from build123d import *

# Parameters (mm, degrees)
BOSS_EXTRUDE1_DEPTH                 = 90
CUT_EXTRUDE1_REACH                  = 116.455
CUT_EXTRUDE2_REACH                  = 116.455
CUT_EXTRUDE2_END_RADIUS             = 50
SKETCH3_W                           = 40
SKETCH3_H                           = 20
CUT_EXTRUDE2_DIRECTION_2_REACH      = 116.455
CUT_EXTRUDE2_DIRECTION_2_END_RADIUS = 50


with BuildPart() as part:
    # Sketch1 → Boss-Extrude1 (new body)
    with BuildSketch(Plane(origin=(0, 0, 0), x_dir=(0, 0, -1), z_dir=(1, 0, 0))):
        with BuildLine():
            Line((-50, 0), (50, 0))
            ThreePointArc((50, 0), (0, 50), (-50, 0))
        make_face()
    extrude(amount=BOSS_EXTRUDE1_DEPTH)

    # Sketch2 → Cut-Extrude1 (cut, up to next)
    with BuildSketch(Plane.ZY, mode=Mode.PRIVATE) as cut_extrude1_sk1:
        Polygon((0, 20.207259422), (-17.5, 10.103629711), (-17.5, -10.103629711), (0, -20.207259422), (17.5, -10.103629711), (17.5, 10.103629711), align=None)
    cut_extrude1_tool1 = extrude(cut_extrude1_sk1.sketch, amount=-CUT_EXTRUDE1_REACH, mode=Mode.PRIVATE) & part.part
    add(cut_extrude1_tool1.solids().sort_by_distance((0, 0, 0))[0], mode=Mode.SUBTRACT)

    # Cut-Extrude2: up to this cylinder (the profile starts inside it)
    cut_extrude2_end = Plane(origin=(45, 0, 0), z_dir=(-1, 0, 0)) * Cylinder(CUT_EXTRUDE2_END_RADIUS, 333.91, mode=Mode.PRIVATE)
    # Sketch3 → Cut-Extrude2 (cut, up to the surface)
    with BuildSketch(Plane.XY, mode=Mode.PRIVATE) as cut_extrude2_sk1:
        with Locations((45, 40)):
            Rectangle(SKETCH3_W, SKETCH3_H)
    cut_extrude2_tool1 = extrude(cut_extrude2_sk1.sketch, amount=-CUT_EXTRUDE2_REACH, mode=Mode.PRIVATE) & cut_extrude2_end
    add(cut_extrude2_tool1.solids().sort_by_distance((45, 40, 0))[0], mode=Mode.SUBTRACT)

    # Cut-Extrude2 direction 2: up to this cylinder (the profile starts inside it)
    cut_extrude2_direction_2_end = Plane(origin=(45, 0, 0), z_dir=(-1, 0, 0)) * Cylinder(CUT_EXTRUDE2_DIRECTION_2_END_RADIUS, 333.91, mode=Mode.PRIVATE)
    # Sketch3 → Cut-Extrude2 direction 2 (cut, up to the surface)
    with BuildSketch(Plane.XY, mode=Mode.PRIVATE) as cut_extrude2_direction_2_sk1:
        with Locations((45, 40)):
            Rectangle(SKETCH3_W, SKETCH3_H)
    cut_extrude2_direction_2_tool1 = extrude(cut_extrude2_direction_2_sk1.sketch, amount=CUT_EXTRUDE2_DIRECTION_2_REACH, mode=Mode.PRIVATE) & cut_extrude2_direction_2_end
    add(cut_extrude2_direction_2_tool1.solids().sort_by_distance((45, 40, 0))[0], mode=Mode.SUBTRACT)


solid = part.part
Verification items for the finished model (mm, model axes). A direction names the side the tool comes from. Round coordinates to 2 decimals unless told otherwise and drop trailing zeros. Loops run counter-clockwise (first coordinate to the right, second up) from the corner with the lowest first, then second, coordinate; pieces in that order, holes last. Notation, with made-up numbers: (-28, -34.5) - (-7, -34.5) arc R27 cw to (-7, 3.5) - close; hole circle Ø8 at (-28, 73). An arc over 180 degrees is marked (long way). Use a Markdown table: item, result. Add a question column.
1. Release check for a two-part mould opening along X. For faces 1 (the face through (0, 25, 1)), 2 (the face through (44.37, 15.226, -8.628)), 3 (the face through (65, 38, 1)) record: released by +X, released by -X, zero draft, split by the parting line, or undercut.
2. Section check A-A, the plane y = 39. Record the boundary of the cut face in (x, z), plus the area to 3 significant figures.
3. Access from +Z, -Z, +X, -X, +Y, -Y to the whole of each face (thin tool, end or side, straight path). Record for faces 4 (the face through (25, 38, 1)), 5 (the face through (44, 0, -34)), 6 (the face through (44.37, 15.085, 8.872)).
4. Thickness scan on probe 1 along X at (y, z) = (40.5, 7); probe 2 along Z at (x, y) = (82, 16); probe 3 along Z at (x, y) = (38.5, 7.5). Record the ranges inside material, lowest first. Write a range as [from, to].
5. Section check D-D, the plane x = 58.5. Record the boundary of the cut face in (y, z), plus the area to 3 significant figures.
6. Section check B-B, the plane x = 8. Record the boundary of the cut face in (y, z).
7. Gauge pin test, flat ends, axial feed: pin 1 (8 mm diameter, centred on x = 31.5, z = -6.5, fed in from +Y); pin 2 (4 mm diameter, centred on x = 25.5, z = -8, fed in from -Y); pin 3 (2 mm diameter, centred on x = 45.5, y = 16, fed in from -Z). Record the tip position at first contact, or that the pin passes through.
8. Section check C-C, the plane z = 12. Record the boundary of the cut face in (x, y), plus the area to 3 significant figures.
Checks:
| question | item | result |
|---|---|---|
| 1 | face 1 | released by -X |
| 1 | face 2 | zero draft |
| 1 | face 3 | undercut |
| 2 | outline | (0, -31.29) - (25, -31.29) - (25, 31.29) - (0, 31.29) - close; (65, -31.29) - (90, -31.29) - (90, 31.29) - (65, 31.29) - close |
| 2 | area | 3,130 mm^2 |
| 3 | face 4 | +Z, -Z, +Y |
| 3 | face 5 | +Z, -Z, +X, -X, -Y |
| 3 | face 6 | +X, -X, -Y |
| 4 | probe 1 | x = [0, 25], [65, 90] |
| 4 | probe 2 | z = [-47.37, -7.29], [7.29, 47.37] |
| 4 | probe 3 | z = [-49.43, -17.5], [17.5, 49.43] |
| 5 | outline | (0, -50) arc R50 ccw to (30, -40) - (30, 40) arc R50 ccw to (0, 50) - (0, 17.5) - (10.1, 17.5) - (20.21, 0) - (10.1, -17.5) - (0, -17.5) - close |
| 5 | area | 2,280 mm^2 |
| 6 | outline | (0, -50) arc R50 ccw to (0, 50) - (0, 17.5) - (10.1, 17.5) - (20.21, 0) - (10.1, -17.5) - (0, -17.5) - close |
| 7 | pin 1 | stops at y = 30 |
| 7 | pin 2 | stops at y = 14.43 |
| 7 | pin 3 | stops at z = -47.7 |
| 8 | outline | (0, 13.28) - (90, 13.28) - (90, 48.54) - (65, 48.54) - (65, 30) - (25, 30) - (25, 48.54) - (0, 48.54) - close |
| 8 | area | 2,430 mm^2 |
